Geometry: final body of the model. Coordinates: model frame, mm. Round coordinates to 2 decimals unless told otherwise and drop trailing zeros. Answer in a Markdown table with one row per item.
```python
from build123d import *

# Parameters (mm, degrees)
SKETCH1_W            = 629.90984
SKETCH1_H            = 147.69846
BOSS_EXTRUDE1_DEPTH  = 3.175
SKETCH3_W            = 254
SKETCH3_H            = 3.175
BOSS_EXTRUDE2_DEPTH  = 6.35
SKETCH4_W            = 3.175
SKETCH4_H            = 188.732840052
CUT_EXTRUDE1_DEPTH   = 3.175
SKETCH6_W            = 3.175
SKETCH6_H            = 110.773845
BOSS_EXTRUDE4_DEPTH  = 3.175
SKETCH8_W            = 629.90984
SKETCH8_H            = 18.04416
BOSS_EXTRUDE5_DEPTH  = 3.175
SKETCH10_W           = 38.1
SKETCH10_H           = 36.08832
CUT_EXTRUDE3_DEPTH   = 652.56536379
BOSS_EXTRUDE6_DEPTH  = 3.175
SKETCH13_R           = 1.55
SKETCH13_R_2         = 11.049
CUT_EXTRUDE4_DEPTH   = 652.56536379
SKETCH20_W           = 20.59499956
SKETCH20_H           = 2.942142794
CUT_EXTRUDE7_DEPTH   = 1.27
SKETCH21_R           = 4.064
CUT_EXTRUDE8_DEPTH   = 652.56536379
SKETCH23_R           = 4.064
CUT_EXTRUDE10_DEPTH  = 652.56536379
M4_CLEARANCE_HOLE1_D = 4.8


with BuildPart() as part:
    # Sketch1 → Boss-Extrude1 (new body)
    with BuildSketch(Plane(origin=(0, 0, 0), x_dir=(1, 0, 0), z_dir=(0, 1, 0))):
        with Locations((314.95492, 73.84923)):
            Rectangle(SKETCH1_W, SKETCH1_H)
    extrude(amount=BOSS_EXTRUDE1_DEPTH)

    # Sketch3 → Boss-Extrude2 (add)
    with BuildSketch(Plane(origin=(0, 0, -147.69846), x_dir=(-1, 0, 0), z_dir=(0, 0, -1))):
        with Locations((-473.22613, 1.5875)):
            Rectangle(SKETCH3_W, SKETCH3_H)
        with Locations((-156.68371, 1.5875)):
            Rectangle(SKETCH3_W, SKETCH3_H)
    extrude(amount=BOSS_EXTRUDE2_DEPTH)

    # Sketch4 → Cut-Extrude1 (cut)
    with BuildSketch(Plane(origin=(0, 3.175, 0), x_dir=(1, 0, 0), z_dir=(0, 1, 0))):
        with Locations((314.95492, 147.69846)):
            Rectangle(SKETCH4_W, SKETCH4_H)
    extrude(amount=-CUT_EXTRUDE1_DEPTH, mode=Mode.SUBTRACT)

    # Sketch6 → Boss-Extrude4 (add)
    with BuildSketch(Plane(origin=(0, 3.175, 0), x_dir=(1, 0, 0), z_dir=(0, 1, 0))):
        with Locations((631.49734, 92.3115375)):
            Rectangle(SKETCH6_W, SKETCH6_H)
        with Locations((-1.5875, 92.3115375)):
            Rectangle(SKETCH6_W, SKETCH6_H)
    extrude(amount=-BOSS_EXTRUDE4_DEPTH)

    # Sketch8 → Boss-Extrude5 (add, through all)
    with BuildSketch(Plane(origin=(0, 3.175, 0), x_dir=(1, 0, 0), z_dir=(0, 1, 0))):
        with Locations((314.95492, -9.02208)):
            Rectangle(SKETCH8_W, SKETCH8_H)
    extrude(amount=-BOSS_EXTRUDE5_DEPTH)

    # Sketch10 → Cut-Extrude3 (cut, through all)
    with BuildSketch(Plane(origin=(0, 3.175, 0), x_dir=(1, 0, 0), z_dir=(0, 1, 0))):
        with Locations((579.10984, -18.04416)):
            Rectangle(SKETCH10_W, SKETCH10_H)
        with Locations((50.8, -18.04416)):
            Rectangle(SKETCH10_W, SKETCH10_H)
    extrude(amount=-CUT_EXTRUDE3_DEPTH, mode=Mode.SUBTRACT)

    # Sketch11 → Boss-Extrude6 (add, through all)
    with BuildSketch(Plane(origin=(0, 3.175, 0), x_dir=(1, 0, 0), z_dir=(0, 1, 0))):
        Polygon((0, -18.04416), (0, -137.42416), (629.90984, -137.42416), (629.90984, -18.04416), (598.15984, -18.04416), (598.15984, -27.06624), (560.05984, -27.06624), (560.05984, -18.04416), (386.39242, -18.04416), (348.29242, -18.04416), (281.61742, -18.04416), (243.51742, -18.04416), (69.85, -18.04416), (69.85, -26.95194), (31.75, -26.95194), (31.75, -18.04416), align=None)
    extrude(amount=-BOSS_EXTRUDE6_DEPTH)

    # Sketch13 → Cut-Extrude4 (cut, through all)
    with BuildSketch(Plane.XZ):
        with Locations(Location((227.731580951, 122.331796051, 0), (0, 0, 270))):
            Circle(SKETCH13_R)
        with Locations(Location((250.731580951, 122.331796051, 0), (0, 0, 270))):
            Circle(SKETCH13_R)
        with Locations(Location((227.731580951, 99.331796051, 0), (0, 0, 270))):
            Circle(SKETCH13_R)
        with Locations(Location((250.731580951, 99.331796051, 0), (0, 0, 270))):
            Circle(SKETCH13_R)
        with Locations(Location((152.328523542, 95.877856055, 0), (0, 0, 270))):
            Circle(SKETCH13_R_2)
        with Locations(Location((227.731580951, 79.083184621, 0), (0, 0, 270))):
            Circle(SKETCH13_R)
        with Locations(Location((227.731580951, 56.083184621, 0), (0, 0, 270))):
            Circle(SKETCH13_R)
        with Locations(Location((250.731580951, 56.083184621, 0), (0, 0, 270))):
            Circle(SKETCH13_R)
        with Locations(Location((250.731580951, 79.083184621, 0), (0, 0, 270))):
            Circle(SKETCH13_R)
        with BuildLine():
            Line((245.043121195, 100.323796051), (233.420040708, 100.323796051))
            ThreePointArc((233.420040708, 100.323796051), (227.223580951, 110.831796051), (233.420040708, 121.339796051))
            Line((233.420040708, 121.339796051), (245.043121195, 121.339796051))
            ThreePointArc((245.043121195, 121.339796051), (251.239580951, 110.831796051), (245.043121195, 100.323796051))
        make_face()
        with BuildLine():
            Line((249.739580951, 73.394724865), (249.739580951, 61.771644378))
            ThreePointArc((249.739580951, 61.771644378), (239.231580951, 55.575184621), (228.723580951, 61.771644378))
            Line((228.723580951, 61.771644378), (228.723580951, 73.394724865))
            ThreePointArc((228.723580951, 73.394724865), (239.231580951, 79.591184621), (249.739580951, 73.394724865))
        make_face()
    extrude(amount=-CUT_EXTRUDE4_DEPTH, mode=Mode.SUBTRACT)

    # Sketch20 → Cut-Extrude7 (cut)
    with BuildSketch(Plane.XZ):
        Polygon((269.946527362, 71.481147903), (278.936408122, 71.481147903), (278.936408122, 69.356266996), (269.946527362, 69.356266996), (269.946527362, 61.837457633), (266.18712268, 61.837457633), (266.18712268, 69.356266996), (258.341408562, 69.356266996), (258.341408562, 71.481147903), (266.18712268, 71.481147903), (266.18712268, 78.999957266), (269.946527362, 78.999957266), align=None)
        with Locations((268.638908342, 111.690432757)):
            Rectangle(SKETCH20_W, SKETCH20_H)
    extrude(amount=-CUT_EXTRUDE7_DEPTH, mode=Mode.SUBTRACT)

    # Sketch21 → Cut-Extrude8 (cut, through all)
    with BuildSketch(Plane(origin=(0, 3.175, 0), x_dir=(1, 0, 0), z_dir=(0, 1, 0))):
        with Locations(Location((168.943513391, -126.78664, 0), (0, 0, 270))):
            Circle(SKETCH21_R)
        with Locations(Location((314.95492, -126.78664, 0), (0, 0, 270))):
            Circle(SKETCH21_R)
        with Locations(Location((460.966326609, -126.78664, 0), (0, 0, 270))):
            Circle(SKETCH21_R)
        with Locations(Location((606.977733219, -126.78664, 0), (0, 0, 270))):
            Circle(SKETCH21_R)
        with Locations(Location((22.932106781, -126.78664, 0), (0, 0, 90))):
            Circle(SKETCH21_R)
    extrude(amount=-CUT_EXTRUDE8_DEPTH, mode=Mode.SUBTRACT)

    # Sketch23 → Cut-Extrude10 (cut, through all)
    with BuildSketch(Plane(origin=(0, 3.175, 0), x_dir=(1, 0, 0), z_dir=(0, 1, 0))):
        with Locations(Location((538.347516778, -9.779, 0), (0, 0, 270))):
            Circle(SKETCH23_R)
        with Locations(Location((375.40565, -9.779, 0), (0, 0, 270))):
            Circle(SKETCH23_R)
        with Locations(Location((254.50419, -9.779, 0), (0, 0, 270))):
            Circle(SKETCH23_R)
        with Locations(Location((91.562323222, -9.779, 0), (0, 0, 270))):
            Circle(SKETCH23_R)
    extrude(amount=-CUT_EXTRUDE10_DEPTH, mode=Mode.SUBTRACT)

    # M4 Clearance Hole1 (through all)
    with Locations(Plane(origin=(0, 3.175, 0), x_dir=(1, 0, 0), z_dir=(0, 1, 0))):
        with Locations((611.402306504, -5.996840051), (510.650895752, -5.996840051), (473.22613, -5.996840051), (435.801364248, -5.996840051), (335.049803495, -5.996840051), (294.860036505, -5.996840051), (194.108475752, -5.996840051), (156.68371, -5.996840051), (119.258944248, -5.996840051), (18.507533496, -5.996840051)):
            Hole(M4_CLEARANCE_HOLE1_D / 2)


solid = part.part
```
Item 1: Cut plane A-A (y = 2.5). Count the separate pieces of the cut face and the enclosed holes in it, then the cut area to 3 significant figures.
Answer:
| item | result |
|---|---|
| separate pieces | 1 |
| enclosed holes | 32 |
| area | 179,000 mm² |
Item 2: Line query: probe 1 along X at (y, z) = (1.85, -84.5) (3 decimals); probe 2 along Z at (x, y) = (563.5, 0.75); probe 3 along X at (y, z) = (1.45, 23.5). Output: solid intervals per line, ascending. Write a range as [from, to].
Answer:
| item | result |
|---|---|
| probe 1 | x = [-3.175, 313.367], [316.542, 633.085] |
| probe 2 | z = [-154.05, 0], [27.07, 137.42] |
| probe 3 | x = [0, 31.75], [69.85, 560.06], [598.16, 629.91] |
Item 3: Pin query (flat end, axial travel): pin 1 Ø1.6 at (y, z) = (2, 71.5) entering from -X; pin 2 Ø10.5 at (x, z) = (538.35, 9.78) entering from -Y; pin 3 Ø1 at (y, z) = (0.5, 74) entering from +X. Return the tip coordinate at first contact, or that it passes through.
Answer:
| item | result |
|---|---|
| pin 1 | stops at x = 0 |
| pin 2 | stops at y = 0 |
| pin 3 | stops at x = 629.91 |
Item 4: Draft query along X for faces 1 (the face through (311, 3.175, -10)), 2 (the face through (163.284, 1.565, 97.316)). Return one class per face: pulls with the +X half, pulls with the -X half, needs draft (parallel to the pull), parting line crosses it, or undercut.
Answer:
| item | result |
|---|---|
| face 1 | needs draft |
| face 2 | undercut |
